Geometry check sheet. Reference: the model listing, model coordinates, mm. Coordinates: 2 decimals unless noted, no trailing zeros. Write each loop counter-clockwise with the first axis right and the second up, starting at its lowest first coordinate (ties: lowest second). Pieces come first, ordered by that corner, then holes. Notation, with made-up numbers: (71.25, -30) - (105.25, -30) arc R12 ccw to (105.25, -23) - close; hole circle Ø6 at (28.5, -3.75). An arc over 180 degrees is marked (long way). Answer as a JSON object with one key per item and string values. Group by question number.
from build123d import *

# Parameters (mm, degrees)
SKETCH1_W            = 60
SKETCH1_H            = 37
BOSS_EXTRUDE1_DEPTH  = 1.5748
FILLET1_R            = 4
SKETCH2_R            = 1.6
CUT_EXTRUDE1_DEPTH   = 36.280731215
SKETCH3_R            = 1.016
CUT_EXTRUDE2_DEPTH   = 36.280731215
SKETCH4_R            = 0.6477
CUT_EXTRUDE3_DEPTH   = 36.280731215
LPATTERN1_COUNT      = 4
LPATTERN1_PITCH      = 5.08
SKETCH5_R            = 0.508
CUT_EXTRUDE4_DEPTH   = 36.280731215
LPATTERN2_COUNT      = 3
LPATTERN2_PITCH      = 2.54
LPATTERN2_COUNT_DIR2 = 2
LPATTERN2_PITCH_DIR2 = 7.62


with BuildPart() as part:
    # Sketch1 → Boss-Extrude1 (new body)
    with BuildSketch(Plane(origin=(0, 0, 0), x_dir=(1, 0, 0), z_dir=(0, 1, 0))):
        Rectangle(SKETCH1_W, SKETCH1_H)
    extrude(amount=BOSS_EXTRUDE1_DEPTH)

    # Fillet1
    fillet1_edges = [part.edges().sort_by_distance(p)[0] for p in [
        (30, 0.7874, 18.5),
        (-30, 0.7874, 18.5),
        (-30, 0.7874, -18.5),
        (30, 0.7874, -18.5),
    ]]
    fillet(fillet1_edges, radius=FILLET1_R)

    # Sketch2 → Cut-Extrude1 (cut, through all)
    with BuildSketch(Plane(origin=(0, 1.5748, 0), x_dir=(1, 0, 0), z_dir=(0, 1, 0))):
        with Locations(Location((-26, 14.5, 0), (0, 0, 270))):
            Circle(SKETCH2_R)
        with Locations(Location((-26, -14.5, 0), (0, 0, 270))):
            Circle(SKETCH2_R)
        with Locations(Location((26, -14.5, 0), (0, 0, 270))):
            Circle(SKETCH2_R)
        with Locations(Location((26, 14.5, 0), (0, 0, 270))):
            Circle(SKETCH2_R)
    extrude(amount=-CUT_EXTRUDE1_DEPTH, mode=Mode.SUBTRACT)

    # Sketch3 → Cut-Extrude2 (cut, through all)
    with BuildSketch(Plane(origin=(0, 1.5748, 0), x_dir=(-1, 0, 0), z_dir=(0, 1, 0))):
        with Locations(Location((4.318, 4.699, 0), (0, 0, 90))):
            Circle(SKETCH3_R)
        with Locations(Location((-17.526, 4.699, 0), (0, 0, 90))):
            Circle(SKETCH3_R)
    extrude(amount=-CUT_EXTRUDE2_DEPTH, mode=Mode.SUBTRACT)

    # Sketch4 → Cut-Extrude3 (cut, through all)
    with BuildSketch(Plane(origin=(0, 1.5748, 0), x_dir=(1, 0, 0), z_dir=(0, 1, 0))):
        with Locations(Location((6.731, -12.319, 0), (0, 0, 270))):
            Circle(SKETCH4_R)
    cut_extrude3 = extrude(amount=-CUT_EXTRUDE3_DEPTH, mode=Mode.SUBTRACT)

    # LPattern1: Cut-Extrude3 ×4
    with Locations(*[(-i * LPATTERN1_PITCH, 0, 0) for i in range(1, LPATTERN1_COUNT)]):
        add(cut_extrude3, mode=Mode.SUBTRACT)

    # Sketch5 → Cut-Extrude4 (cut, through all)
    with BuildSketch(Plane(origin=(0, 1.5748, 0), x_dir=(1, 0, 0), z_dir=(0, 1, 0))):
        with Locations(Location((-13.589, -14.478, 0), (0, 0, 270))):
            Circle(SKETCH5_R)
    cut_extrude4 = extrude(amount=-CUT_EXTRUDE4_DEPTH, mode=Mode.SUBTRACT)

    # LPattern2: Cut-Extrude4 3 × 2
    with Locations(*[(-i * LPATTERN2_PITCH, 0, -j * LPATTERN2_PITCH_DIR2) for i in range(LPATTERN2_COUNT) for j in range(LPATTERN2_COUNT_DIR2) if (i, j) != (0, 0)]):
        add(cut_extrude4, mode=Mode.SUBTRACT)


solid = part.part
(1) Section check B-B (y = 1.05). Count the separate pieces of the cut face and the enclosed holes in it, and give its area (3 significant figures).
(2) Section check A-A (z = -15.5). Record the cut outline in (x, y), and give its area (3 significant figures).
(3) Material ranges on L1, parallel to X at y = 0.75, z = 14.5; L2, parallel to X at y = 1.1, z = -15.5; L3, parallel to X at y = 0.45, z = 5, recorded low to high. Write a range as [from, to].
(4) Draft check along Z on faces 1 (the face through (7.373, 0.798, 12.235)), 2 (the face through (27.08, 0.8, 13.32)), 3 (the face through (0, 1, -18.5)), 4 (the face through (0, 0, 0)). Enter one of: +Z half, -Z half, draft (parallel to the pull), parting line (faces both ways), or undercut.
Conclusion:
{
 "1": {"separate pieces": "1", "enclosed holes": "16", "area": "2,160 mm^2"},
 "2": {"outline": "(-29.87, 0) - (-27.25, 0) - (-27.25, 1.57) - (-29.87, 1.57) - close; (-24.75, 0) - (24.75, 0) - (24.75, 1.57) - (-24.75, 1.57) - close; (27.25, 0) - (29.87, 0) - (29.87, 1.57) - (27.25, 1.57) - close", "area": "86.2 mm^2"},
 "3": {"L1": "x = [-30, -27.6], [-24.4, -19.18], [-18.16, -16.64], [-15.62, -14.1], [-13.08, 24.4], [27.6, 30]", "L2": "x = [-29.87, -27.25], [-24.75, 24.75], [27.25, 29.87]", "L3": "x = [-30, -5.29], [-3.35, 16.56], [18.5, 30]"},
 "4": {"face 1": "undercut", "face 2": "undercut", "face 3": "-Z half", "face 4": "draft"}
}
